Autodesk Inventor part; units mm, degrees
ref_plane "YZ Plane" through (0, 0, 0) normal (1, 0, 0) x (0, 1, 0)
ref_plane "XZ Plane" through (0, 0, 0) normal (0, 1, 0) x (-1, 0, 0)
ref_plane "XY Plane" through (0, 0, 0) normal (0, 0, 1) x (1, 0, 0)
sketch "Sketch1" plane through (0, 0, 0) normal (0, 0, 1) x (1, 0, 0)
  circle A0 centre (0, 0) radius 1625.6
  circle A1 centre (0, 0) radius 32
  line L0 (0, 32) -> (0, -32) construction
  line L1 (-32, 0) -> (32, 0) construction
  dimension "d2" = 64
extrude "Extrusion1" add sketch "Sketch1" along normal blind 18 contours A1
sketch "Sketch2" plane through (0, 0, 18) normal (0, 0, 1) x (1, 0, 0)
  circle A0 centre (0, 0) radius 10.5
  dimension "d7" = 21
extrude "Extrusion2" add sketch "Sketch2" along normal blind 21
sketch "Sketch3" plane through (0, 0, 39) normal (0, 0, 1) x (1, 0, 0)
  circle A0 centre (0, 0) radius 7.5
  dimension "d10" = 15
extrude "Extrusion3" add sketch "Sketch3" along normal blind 11
sketch "Sketch4" plane through (0, 0, 50) normal (0, 0, 1) x (1, 0, 0)
  circle A0 centre (0, 0) radius 5
  dimension "d13" = 10
extrude "Extrusion4" add sketch "Sketch4" along normal blind 20
sketch "Sketch5" plane through (0, 0, 70) normal (0, 0, 1) x (1, 0, 0)
  circle A0 centre (0, 0) radius 4
  dimension "d16" = 8
extrude "Extrusion5" add sketch "Sketch5" along normal blind 14
sketch "Sketch6" plane through (0, 0, 84) normal (0, 0, 1) x (1, 0, 0)
  circle A0 centre (0, 0) radius 5
  dimension "d19" = 10
extrude "Extrusion6" add sketch "Sketch6" along normal blind 32
Could you check a few things on this model? Use its own coordinates, in mm. Round coordinates to 2 decimals unless told otherwise and drop trailing zeros. Order: outer loops, then holes, each group sorted by start corner. A loop starts at its lowest first (then second) coordinate and runs counter-clockwise, first axis right, second up.
Q1. Imagine slicing it at C-C, the plane z = 99. List the corners of the cut face in (x, y) for me.
Geometry says:
outline: circle Ø10 at (0, 0)
Q2. Imagine slicing it at D-D, the plane z = 80.5. List the corners of the cut face in (x, y) for me, then the cut area to 3 significant figures.
Geometry says:
outline: circle Ø8 at (0, 0)
area: 50.3 mm2
Q3. Imagine slicing it at A-A, the plane y = 0. List the corners of the cut face in (x, z) for me, then the cut area to 3 significant figures.
Geometry says:
outline: (-32, 0) - (32, 0) - (32, 18) - (10.5, 18) - (10.5, 39) - (7.5, 39) - (7.5, 50) - (5, 50) - (5, 70) - (4, 70) - (4, 84) - (5, 84) - (5, 116) - (-5, 116) - (-5, 84) - (-4, 84) - (-4, 70) - (-5, 70) - (-5, 50) - (-7.5, 50) - (-7.5, 39) - (-10.5, 39) - (-10.5, 18) - (-32, 18) - close
area: 2,390 mm2
Q4. Please list where these lines run through material, in increasing order: probe 1 along Z at (x, y) = (-3.5, -28); probe 2 along Y at (x, z) = (-3, 97.5); probe 3 along Z at (x, y) = (-3.5, 5).
Geometry says:
probe 1: z = 0 to 18
probe 2: y = -4 to 4
probe 3: z = 0 to 50
Q5. I'm going to push flat-ended pins straight in: P1, Ø5, axis at x = 0.5, y = 18, coming from the +Z side; P2, Ø6, axis at x = 5.5, y = 9.5, coming from the +Z side; P3, Ø5, axis at y = 1.5, z = 103.5, coming from the -X side. Where does each tip first touch, or does it pass through?
Geometry says:
P1: stops at z = 18
P2: stops at z = 39
P3: stops at x = -5
Q6. Thinking about a two-plate mould opening in Z: for faces 1 (the face through (-6.94, 31.24, 8.87)), 2 (the face through (0, 0, 0)), 3 (the face through (-0.867, 3.905, 76.902)), 4 (the face through (0, 0, 116)), which applies, released by +Z, released by -Z, zero draft, split by the parting line, or undercut?
Geometry says:
face 1: zero draft
face 2: released by -Z
face 3: undercut
face 4: released by +Z
